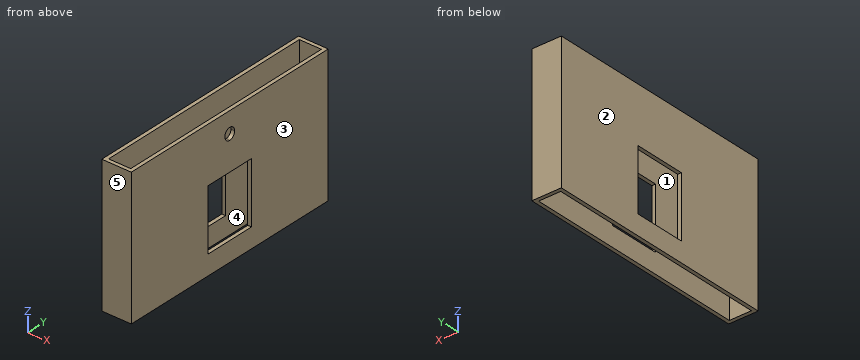
from build123d import *

# Parameters (mm, degrees)
F0_W     = 152.4
F0_H     = 1212.85
F0_W_2   = 114.3
F0_H_2   = 1174.75
F1_DEPTH = 704.85
F3_DEPTH = 25.4
F5_DEPTH = 19.05


# Not quite as in the source:
# - a feature names something its author has since deleted; it is built from what else it names


with BuildPart() as f1:
    # F0 (on Top) → F1 (new body)
    with BuildSketch(Plane.XY):
        Rectangle(F0_W, F0_H)
        Rectangle(F0_W_2, F0_H_2, mode=Mode.SUBTRACT)
    extrude(amount=F1_DEPTH)

    # F2 (on face) → F3 (cut)
    with BuildSketch(Plane.YZ.offset(76.2)):
        with BuildLine():
            ThreePointArc((30.226, 596.9), (-21.3730095681, 618.2730095681), (0, 566.674))
            ThreePointArc((0, 566.674), (21.3730095681, 575.5269904319), (30.226, 596.9))
        make_face()
        Polygon((-133.35, 101.6), (0, 101.6), (133.35, 101.6), (133.35, 419.1), (0, 419.1), (-133.35, 419.1), align=None)
    extrude(amount=-F3_DEPTH, mode=Mode.SUBTRACT)

    # F4 (on face) → F5 (cut)
    with BuildSketch(Plane(origin=(-76.2, 0, 0), x_dir=(0, -1, 0), z_dir=(-1, 0, 0))):
        Polygon((-133.35, 101.6), (0, 101.6), (133.35, 101.6), (133.35, 419.1), (-133.35, 419.1), align=None)
    extrude(amount=-F5_DEPTH, mode=Mode.SUBTRACT)


solid = f1.part
Source: CAD feature listing. Evaluate the final solid. Frame: model axes, mm. Face numbers are marked on the shaded views. A direction names the side the tool comes from. Give positions to 0.01 mm unless a question says otherwise; leave off trailing zeros. Write each loop counter-clockwise with the first axis right and the second up, starting at its lowest first coordinate (ties: lowest second). Pieces come first, ordered by that corner, then holes. Notation, with made-up numbers: (-13, -27.75) - (34, -27.75) arc R24 ccw to (34, -12.75) - close; hole circle Ø4 at (8.5, 11). An arc over 180 degrees is marked (long way). Write item = value, one per line. Start each with the question number.
Q1. Pin query (flat end, axial travel): pin 1 Ø5.5 at (x, y) = (-63, -5.5) entering from -Z; pin 2 Ø10 at (x, y) = (-49, 109) entering from +Z. Return the tip coordinate at first contact, or that it passes through.
Q2. Cut plane D-D, the plane y = -274. Return loops of the section in (x, z), then the cut area to 3 significant figures.
Q3. Reachability of the marked faces 1 and 2 from +Z, -Z, +X, -X, +Y, -Y: full face, straight path, thin tool, end or side. Return the list, or none.
Q4. Cut plane C-C, the plane x = 23. Return loops of the section in (y, z) (3 decimals), then the cut area to 3 significant figures.
Q5. Cut plane B-B, the plane y = 55. Return loops of the section in (x, z), then the cut area to 3 significant figures.
Q6. Material intervals for probe 1 along Z at (x, y) = (67.25, 0); probe 2 along X at (y, z) = (-537.5, 144); probe 3 along Y at (x, z) = (70, 596) (3 decimals), sorted ascending.
Q7. Cut plane A-A, the plane z = 58.5. Return loops of the section in (x, y) (3 decimals).
Q8. Draft query along X for the marked faces 3, 4 and 5. Return one class per face: +X half, -X half, draft (parallel to the pull), parting line (faces both ways), or undercut.
Computed values:
q1.pin_1 = 0
q1.pin_2 = through
q2.outline = (-76.2, 0) - (-57.15, 0) - (-57.15, 704.85) - (-76.2, 704.85) - close; (57.15, 0) - (76.2, 0) - (76.2, 704.85) - (57.15, 704.85) - close
q2.area = 26,900 mm²
q3.face_1 = +Z, -Z
q3.face_2 = +Z, -Z, -X, +Y, -Y
q4.outline = (-606.425, 0) - (-587.375, 0) - (-587.375, 704.85) - (-606.425, 704.85) - close; (587.375, 0) - (606.425, 0) - (606.425, 704.85) - (587.375, 704.85) - close
q4.area = 26,900 mm²
q5.outline = (-76.2, 0) - (-57.15, 0) - (-57.15, 101.6) - (-76.2, 101.6) - close; (-76.2, 419.1) - (-57.15, 419.1) - (-57.15, 704.85) - (-76.2, 704.85) - close; (57.15, 0) - (76.2, 0) - (76.2, 101.6) - (57.15, 101.6) - close; (57.15, 419.1) - (76.2, 419.1) - (76.2, 704.85) - (57.15, 704.85) - close
q5.area = 14,800 mm²
q6.probe_1 = 0 to 101.6, 419.1 to 566.67, 627.13 to 704.85
q6.probe_2 = -76.2 to -57.15, 57.15 to 76.2
q6.probe_3 = -606.425 to -30.213, 30.213 to 606.425
q7.outline = (-76.2, -606.425) - (76.2, -606.425) - (76.2, 606.425) - (-76.2, 606.425) - close; hole (-57.15, -587.375) - (57.15, -587.375) - (57.15, 587.375) - (-57.15, 587.375) - close
q8.face_3 = +X half
q8.face_4 = undercut
q8.face_5 = draft
